```python
from build123d import *

# Parameters (mm, degrees)
SKETCH1_R           = 44
BOSS_EXTRUDE1_DEPTH = 180
SKETCH7_R           = 39.5
CUT_EXTRUDE1_DEPTH  = 115
SKETCH8_R           = 35
CUT_EXTRUDE2_DEPTH  = 18
SKETCH12_W          = 11.2
SKETCH12_H          = 156.702496638
CUT_EXTRUDE5_DEPTH  = 13.6
SKETCH14_W          = 11.2
SKETCH14_H          = 8.676367157
CUT_EXTRUDE6_DEPTH  = 18
SKETCH18_R          = 39.5
CUT_EXTRUDE8_DEPTH  = 12
CUT_EXTRUDE4_DEPTH  = 21
CUT_EXTRUDE9_DEPTH  = 28
SKETCH21_R          = 44
CUT_EXTRUDE10_DEPTH = 10
CUT_EXTRUDE11_DEPTH = 50
SKETCH24_R          = 10
CUT_EXTRUDE12_DEPTH = 16
SKETCH26_W          = 11.2
SKETCH26_H          = 11
CUT_EXTRUDE13_DEPTH = 14
SKETCH27_R          = 39
CUT_EXTRUDE14_DEPTH = 30
SKETCH28_R          = 47
SKETCH28_R_2        = 42
BOSS_EXTRUDE2_DEPTH = 20
CUT_EXTRUDE15_DEPTH = 40
SKETCH30_R          = 47
CUT_EXTRUDE16_DEPTH = 20
SKETCH33_R          = 44
CUT_EXTRUDE17_DEPTH = 137
BOSS_EXTRUDE4_DEPTH = 5
SKETCH35_W          = 70
SKETCH35_H          = 2
CUT_EXTRUDE18_DEPTH = 5
SKETCH37_R          = 44
CUT_EXTRUDE19_DEPTH = 9
CUT_EXTRUDE20_DEPTH = 5


with BuildPart() as part:
    # Sketch1 → Boss-Extrude1 (new body)
    with BuildSketch(Plane(origin=(0, 0, 0), x_dir=(1, 0, 0), z_dir=(0, 1, 0))):
        Circle(SKETCH1_R)
    extrude(amount=BOSS_EXTRUDE1_DEPTH)

    # Sketch7 → Cut-Extrude1 (cut)
    with BuildSketch(Plane(origin=(0, 25, 0), x_dir=(1, 0, 0), z_dir=(0, 1, 0))):
        Circle(SKETCH7_R)
    extrude(amount=CUT_EXTRUDE1_DEPTH, mode=Mode.SUBTRACT)

    # Sketch8 → Cut-Extrude2 (cut)
    with BuildSketch(Plane(origin=(0, 41, 0), x_dir=(1, 0, 0), z_dir=(0, 1, 0))):
        Circle(SKETCH8_R)
    extrude(amount=-CUT_EXTRUDE2_DEPTH, mode=Mode.SUBTRACT)

    # Sketch12 → Cut-Extrude5 (cut)
    with BuildSketch(Plane.XY.offset(42)):
        with Locations((0, 88.648751681)):
            Rectangle(SKETCH12_W, SKETCH12_H)
    extrude(amount=CUT_EXTRUDE5_DEPTH, mode=Mode.SUBTRACT)

    # Sketch14 → Cut-Extrude6 (cut)
    with BuildSketch(Plane.XY.offset(42)):
        with Locations((0, 14.635686941)):
            Rectangle(SKETCH14_W, SKETCH14_H)
    extrude(amount=-CUT_EXTRUDE6_DEPTH, mode=Mode.SUBTRACT)

    # Sketch18 → Cut-Extrude8 (cut)
    with BuildSketch(Plane(origin=(0, 180, 0), x_dir=(1, 0, 0), z_dir=(0, 1, 0))):
        Circle(SKETCH18_R)
    extrude(amount=-CUT_EXTRUDE8_DEPTH, mode=Mode.SUBTRACT)

    # Sketch10 → Cut-Extrude4 (cut, symmetric)
    with BuildSketch(Plane(origin=(0, 174, 0), x_dir=(1, 0, 0), z_dir=(0, 1, 0))):
        with BuildLine():
            Line((-39.5, 0), (39.5, 0))
            ThreePointArc((39.5, 0), (0, -39.5), (-39.5, 0))
        make_face()
    extrude(amount=CUT_EXTRUDE4_DEPTH, both=True, mode=Mode.SUBTRACT)

    # Sketch20 → Cut-Extrude9 (cut)
    with BuildSketch(Plane(origin=(0, 168, 0), x_dir=(1, 0, 0), z_dir=(0, 1, 0))):
        with BuildLine():
            Line((9, 26), (-15, 26))
            ThreePointArc((-15, 26), (-18.535533906, 24.535533906), (-20, 21))
            Line((-20, 21), (-20, 10))
            ThreePointArc((-20, 10), (-18.535533906, 6.464466094), (-15, 5))
            Line((-15, 5), (9, 5))
            ThreePointArc((9, 5), (12.535533906, 6.464466094), (14, 10))
            Line((14, 10), (14, 21))
            ThreePointArc((14, 21), (12.535533906, 24.535533906), (9, 26))
        make_face()
    extrude(amount=-CUT_EXTRUDE9_DEPTH, mode=Mode.SUBTRACT)

    # Sketch21 → Cut-Extrude10 (cut)
    with BuildSketch(Plane(origin=(0, 5, 0), x_dir=(1, 0, 0), z_dir=(0, 1, 0))):
        Circle(SKETCH21_R)
    extrude(amount=-CUT_EXTRUDE10_DEPTH, mode=Mode.SUBTRACT)

    # Sketch23 → Cut-Extrude11 (cut)
    with BuildSketch(Plane(origin=(0, 168, 0), x_dir=(1, 0, 0), z_dir=(0, 1, 0))):
        with BuildLine():
            Line((-34.700571143, 4.568409172), (34.700571143, 4.568409172))
            ThreePointArc((34.700571143, 4.568409172), (0, 35), (-34.700571143, 4.568409172))
        make_face()
    extrude(amount=-CUT_EXTRUDE11_DEPTH, mode=Mode.SUBTRACT)

    # Sketch24 → Cut-Extrude12 (cut)
    with BuildSketch(Plane(origin=(0, 153, 0), x_dir=(1, 0, 0), z_dir=(0, 1, 0))):
        with Locations((-17, -14)):
            Circle(SKETCH24_R)
        with Locations((17, -14)):
            Circle(SKETCH24_R)
    extrude(amount=-CUT_EXTRUDE12_DEPTH, mode=Mode.SUBTRACT)

    # Sketch26 → Cut-Extrude13 (cut)
    with BuildSketch(Plane.XY.offset(42)):
        with Locations((0, 161.5)):
            Rectangle(SKETCH26_W, SKETCH26_H)
    extrude(amount=-CUT_EXTRUDE13_DEPTH, mode=Mode.SUBTRACT)

    # Sketch27 → Cut-Extrude14 (cut)
    with BuildSketch(Plane.XZ.offset(-5)):
        Circle(SKETCH27_R)
    extrude(amount=-CUT_EXTRUDE14_DEPTH, mode=Mode.SUBTRACT)

    # Sketch28 → Boss-Extrude2 (add)
    with BuildSketch(Plane.XZ.offset(-5)):
        Circle(SKETCH28_R)
        Circle(SKETCH28_R_2, mode=Mode.SUBTRACT)
    extrude(amount=BOSS_EXTRUDE2_DEPTH)

    # Sketch29 → Cut-Extrude15 (cut)
    with BuildSketch(Plane(origin=(0, 168, 0), x_dir=(1, 0, 0), z_dir=(0, 1, 0))):
        with BuildLine():
            Line((-39.234928796, 4.568409172), (-34.700571143, 4.568409172))
            ThreePointArc((-34.700571143, 4.568409172), (0, 35), (34.700571143, 4.568409172))
            Line((34.700571143, 4.568409172), (39.234928796, 4.568409172))
            ThreePointArc((39.234928796, 4.568409172), (0, 39.5), (-39.234928796, 4.568409172))
        make_face()
    extrude(amount=-CUT_EXTRUDE15_DEPTH, mode=Mode.SUBTRACT)

    # Sketch30 → Cut-Extrude16 (cut)
    with BuildSketch(Plane.XZ.offset(15)):
        Circle(SKETCH30_R)
    extrude(amount=-CUT_EXTRUDE16_DEPTH, mode=Mode.SUBTRACT)

    # Sketch33 → Cut-Extrude17 (cut, through all)
    with BuildSketch(Plane(origin=(0, 141, 0), x_dir=(1, 0, 0), z_dir=(0, 1, 0))):
        Circle(SKETCH33_R)
    extrude(amount=-CUT_EXTRUDE17_DEPTH, mode=Mode.SUBTRACT)

    # Sketch34 → Boss-Extrude4 (add)
    with BuildSketch(Plane.XZ.offset(-141)):
        with BuildLine():
            Line((15.246488352, 37.736382881), (15.845858901, 39.219877048))
            ThreePointArc((15.845858901, 39.219877048), (0, -42.3), (-15.845858901, 39.219877048))
            Line((-15.845858901, 39.219877048), (-15.246488352, 37.736382881))
            ThreePointArc((-15.246488352, 37.736382881), (0, -40.7), (15.246488352, 37.736382881))
        make_face()
    extrude(amount=BOSS_EXTRUDE4_DEPTH)

    # Sketch35 → Cut-Extrude18 (cut)
    with BuildSketch(Plane(origin=(0, 168, 0), x_dir=(1, 0, 0), z_dir=(0, 1, 0))):
        with Locations((0, 2.268409172)):
            Rectangle(SKETCH35_W, SKETCH35_H)
    extrude(amount=-CUT_EXTRUDE18_DEPTH, mode=Mode.SUBTRACT)

    # Sketch37 → Cut-Extrude19 (cut)
    with BuildSketch(Plane(origin=(0, 180, 0), x_dir=(1, 0, 0), z_dir=(0, 1, 0))):
        Circle(SKETCH37_R)
    extrude(amount=-CUT_EXTRUDE19_DEPTH, mode=Mode.SUBTRACT)

    # Sketch38 → Cut-Extrude20 (cut)
    with BuildSketch(Plane(origin=(0, 171, 0), x_dir=(1, 0, 0), z_dir=(0, 1, 0))):
        with BuildLine():
            Line((-14.535856091, -39.936936383), (-13.851815805, -38.057551142))
            ThreePointArc((-13.851815805, -38.057551142), (0, 40.5), (13.851815805, -38.057551142))
            Line((13.851815805, -38.057551142), (14.535856091, -39.936936383))
            ThreePointArc((14.535856091, -39.936936383), (0, 42.5), (-14.535856091, -39.936936383))
        make_face()
    extrude(amount=-CUT_EXTRUDE20_DEPTH, mode=Mode.SUBTRACT)


solid = part.part
```
Check sheet for the modelled part. Datum: model origin and axes. Units: mm. A direction names the side the tool comes from. Coordinates: 2 decimals unless noted, no trailing zeros. Order: outer loops, then holes, each group sorted by start corner. A loop starts at its lowest first (then second) coordinate and runs counter-clockwise, first axis right, second up. Notation, with made-up numbers: (-18, 12) -> (17, 12) arc R26 cw to (17, 30) -> close; hole circle Ø11 at (84.25, 0.5). An arc over 180 degrees is marked (long way). Write item = value, one per line. Start each with the question number.
1) Mould release check, pull along X, two halves, no side actions. Record for faces 5 (the flat face through (-1, 141, 9)), 6 (the cylindrical face through (-9.538, 155.79, 42.954)), 7 (the cylindrical face through (-1.57, 138.54, -40.67)): +X half, -X half, draft (parallel to the pull), parting line (faces both ways), or undercut.
2) Access from +Z, -Z, +X, -X, +Y, -Y to the whole of each face (thin tool, end or side, straight path). Record for faces 1 (the cylindrical face through (1.63, 138.54, -42.27)), 2 (the flat face through (-35, 166, -2)), 3 (the flat face through (-1, 155, -4.568)), 4 (the flat face through (0, 167, 42)).
3) Cross-section at A-A (x = 0). Enter the section's corners in (y, z), then the cut area to 3 significant figures.
4) Material ranges on L1, parallel to Z at x = 0, y = 168.6; L2, parallel to Z at x = 0, y = 165; L3, parallel to X at y = 139, z = 0, recorded low to high.
5) Cross-section at C-C (z = 14). State how many separate pieces and enclosed holes the cut face has, then the cut area to 3 significant figures.
6) Go/stop test with flat-tipped pins: P1, Ø2, axis at y = 162.5, z = 32.5, coming from the +X side; P2, Ø2, axis at y = 165.5, z = -3.5, coming from the +X side; P3, Ø4, axis at x = 1.5, y = 165.5, coming from the +Z side. Record where each tip stops, or that it passes through.
7) Cross-section at B-B (z = -25). Enter the section's corners in (x, y).
Ans:
q1.face_5 = undercut
q1.face_6 = parting line
q1.face_7 = undercut
q2.face_1 = -Y
q2.face_2 = +Y
q2.face_3 = +Y, -Y
q2.face_4 = +Z
q3.outline = (136, -42.3) -> (141, -42.3) -> (141, -44) -> (171, -44) -> (171, -42.5) -> (166, -42.5) -> (166, -40.5) -> (171, -40.5) -> (171, -39.5) -> (141, -39.5) -> (141, -40.7) -> (136, -40.7) -> close; (141, -4.57) -> (168, -4.57) -> (168, -3.27) -> (163, -3.27) -> (163, -1.27) -> (168, -1.27) -> (168, 0) -> (153, 0) -> (153, 39.5) -> (156, 39.5) -> (156, 42) -> (141, 42) -> close; (167, 39.5) -> (171, 39.5) -> (171, 44) -> (167, 44) -> close
q3.area = 776 mm²
q4.L1 = -44 to -42.5, -40.5 to -39.5, 39.5 to 44
q4.L2 = -44 to -39.5, -4.57 to -3.27, -1.27 to 0
q4.L3 = -42.3 to -40.7, 40.7 to 42.3
q5.separate_pieces = 3
q5.enclosed_holes = 0
q5.area = 689 mm²
q6.P1 = 30.72
q6.P2 = 43.93
q6.P3 = 44
q7.outline = (-36.21, 141) -> (-34.12, 141) -> (-34.12, 136) -> (-32.12, 136) -> (-32.12, 141) -> (-30.58, 141) -> (-30.58, 171) -> (-31.86, 171) -> (-31.86, 166) -> (-34.37, 166) -> (-34.37, 171) -> (-36.21, 171) -> close; (30.58, 141) -> (32.12, 141) -> (32.12, 136) -> (34.12, 136) -> (34.12, 141) -> (36.21, 141) -> (36.21, 171) -> (34.37, 171) -> (34.37, 166) -> (31.86, 166) -> (31.86, 171) -> (30.58, 171) -> close
